Verification items for the finished model (mm, model axes). Give positions to 0.01 mm unless a question says otherwise; leave off trailing zeros. Put each result on its own line as item: value.
from build123d import *

# Parameters (mm, degrees)
SKETCH_1_R      = 2.5
SKETCH_1_R_2    = 5
SKETCH_1_R_3    = 1
EXTRUDE_1_DEPTH = 1


with BuildPart() as part:
    # Эскиз1 → Бобышка-Вытянуть1 (new body)
    with BuildSketch(Plane.XY):
        with BuildLine():
            Line((-5.644333703, 13.897551295), (-22.8125, 6.952686082))
            ThreePointArc((-22.8125, 6.952686082), (-27.5, 0), (-22.8125, -6.952686082))
            Line((-22.8125, -6.952686082), (-5.625, -13.905372163))
            ThreePointArc((-5.625, -13.905372163), (-2.865258937, -14.723800162), (0, -15))
            Line((0, -15), (130, -15))
            Line((130, -15), (130, 15))
            Line((130, 15), (0, 15))
            ThreePointArc((0, 15), (-2.875496154, 14.721811827), (-5.644333703, 13.897551295))
        make_face()
        with Locations((-20, 0)):
            Circle(SKETCH_1_R, mode=Mode.SUBTRACT)
        with Locations((-3.8531e-05, 0)):
            Circle(SKETCH_1_R_2, mode=Mode.SUBTRACT)
        with Locations((25, 12)):
            Circle(SKETCH_1_R_3, mode=Mode.SUBTRACT)
        with Locations((50, 12)):
            Circle(SKETCH_1_R_3, mode=Mode.SUBTRACT)
        with Locations((75, 12)):
            Circle(SKETCH_1_R_3, mode=Mode.SUBTRACT)
        with Locations((100, 12)):
            Circle(SKETCH_1_R_3, mode=Mode.SUBTRACT)
        with Locations((25, -12)):
            Circle(SKETCH_1_R_3, mode=Mode.SUBTRACT)
        with Locations((50, -12)):
            Circle(SKETCH_1_R_3, mode=Mode.SUBTRACT)
        with Locations((75, -12)):
            Circle(SKETCH_1_R_3, mode=Mode.SUBTRACT)
        with Locations((100, -12)):
            Circle(SKETCH_1_R_3, mode=Mode.SUBTRACT)
    extrude(amount=EXTRUDE_1_DEPTH)


solid = part.part
Q1. Release check for a two-part mould opening along Y. For faces 1 (the face through (-27.5, 0.1, 0.5)), 2 (the face through (-14.34, -10.38, 0.49)), 3 (the face through (-14.108, 10.474, 0.493)), 4 (the face through (4.77, 1.5, 0.49)) record: released by +Y, released by -Y, zero draft, split by the parting line, or undercut.
Answers follow:
face 1: split by the parting line
face 2: released by -Y
face 3: released by +Y
face 4: undercut
Q2. Scan lines: line 1 along Y through (x, z) = (50, 0.65); line 2 along X through (y, z) = (8, 0.2); line 3 along X through (y, z) = (5.5, 0.95). Record each from-to range of solid material in increasing order.
Answers follow:
line 1: y = -15 to -13, -11 to 11, 13 to 15
line 2: x = -20.22 to 130
line 3: x = -25.1 to 130
Q3. Section check A-A, the plane z = 0.35. Give the number of separate pieces and of enclosed holes in the cut face, plus the area to 3 significant figures.
Answers follow:
separate pieces: 1
enclosed holes: 10
area: 4,350 mm2
Q4. Go/stop test with a flat-tipped pin: pin 1 Ø1.6 at (x, y) = (75, 12) entering from -Z. Record where the tip stops, or that it passes through.
Answers follow:
pin 1: passes through
